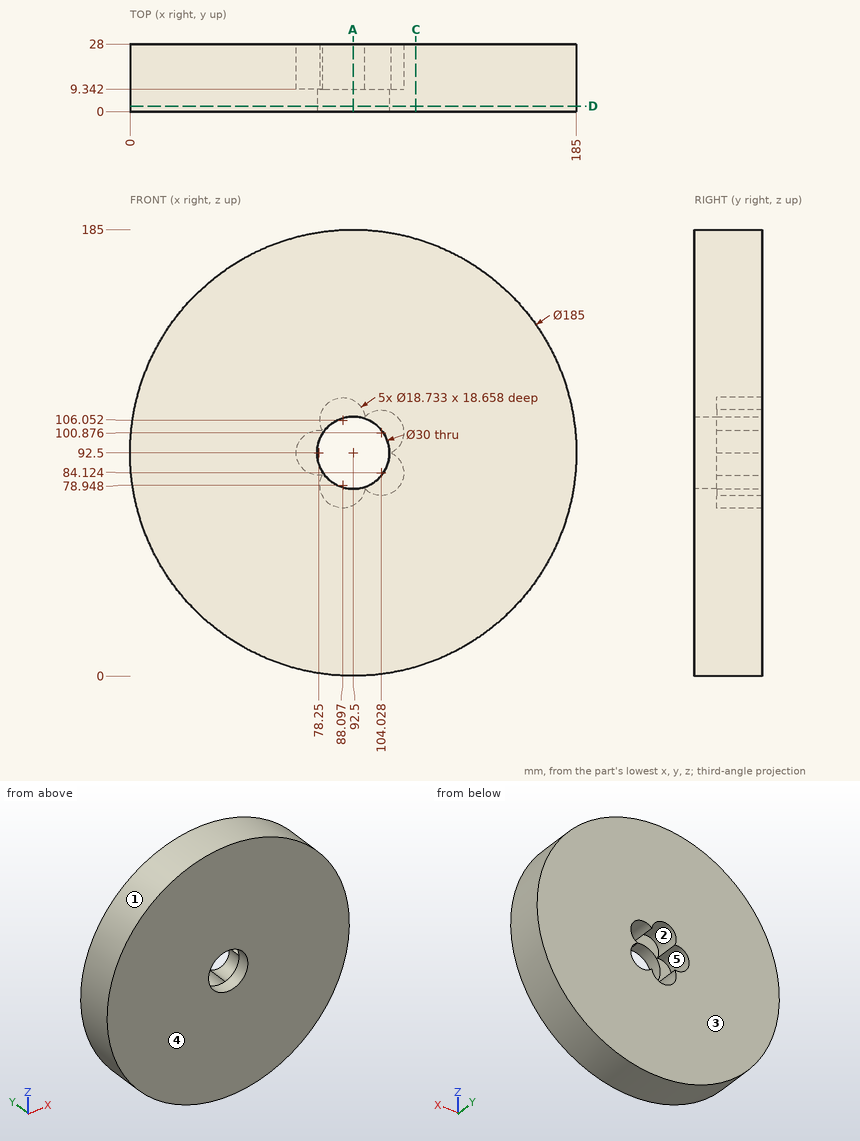
Design review of the part shown in the three views and the two pictorial views. Dimensions are in mm from the part's minimum x, y and z. A direction names the side the tool comes from. Coordinates: 2 decimals unless noted, no trailing zeros. Write each loop counter-clockwise with the first axis right and the second up, starting at its lowest first coordinate (ties: lowest second). Pieces come first, ordered by that corner, then holes.
1) We need section A-A on x = 92.5. State the section outline as (y, z) points, then the cut area to 3 significant figures.
2) We need section D-D on y = 2.25. State the section outline as (x, z) points, then the cut area to 3 significant figures.
3) To check wall thickness, follow probe 1 along X at (y, z) = (2.25, 92.5); probe 2 along X at (y, z) = (5, 97); probe 3 along X at (y, z) = (25.75, 18.5). State the ranges of each line that lie inside material, in increasing order.
4) Clearance check with flat-ended pins moving along their axes: pin 1 Ø3 at (x, z) = (101, 126.5) entering from -Y; pin 2 Ø12 at (x, y) = (159.5, 10) entering from +Z (1 decimal); pin 3 Ø6 at (x, y) = (77, 6) entering from -Z; pin 4 Ø15 at (x, z) = (104.03, 84.12) entering from +Y. State where each tip first meets the part, or that it passes through.
5) We need section C-C on x = 118.5. State the section outline as (y, z) points.
6) Machinability: for the marked faces 4 and 5, which of the approach directions +Z, -Z, +X, -X, +Y, -Y give a long, thin tool a straight path to every point of the face, cutting with its end or side? Answer none if there is none.
7) The part is to be moulded in two halves that separate along X. For the marked faces 1, 2 and 3, say which applies: pulls with the +X half, pulls with the -X half, needs draft (parallel to the pull), parting line crosses it, or undercut.
Answer list:
1. outline: (0, 0) - (28, 0) - (28, 70.68) - (9.34, 70.68) - (9.34, 77.5) - (0, 77.5) - close; (0, 107.5) - (9.34, 107.5) - (9.34, 114.32) - (28, 114.32) - (28, 185) - (0, 185) - close
1. area: 4,090 mm2
2. outline: circle Ø185 at (92.5, 92.5); hole circle Ø30 at (92.5, 92.5)
2. area: 26,200 mm2
3. probe 1: x = 0 to 77.5, 107.5 to 185
3. probe 2: x = 0.11 to 78.19, 106.81 to 184.89
3. probe 3: x = 37 to 148
4. pin 1: stops at y = 0
4. pin 2: stops at z = 162
4. pin 3: stops at z = 0.85
4. pin 4: stops at y = 9.34
5. outline: (0, 3.73) - (28, 3.73) - (28, 181.27) - (0, 181.27) - close
6. face 4: +Z, -Z, +X, -X, -Y
6. face 5: +Y
7. face 1: parting line crosses it
7. face 2: undercut
7. face 3: needs draft
